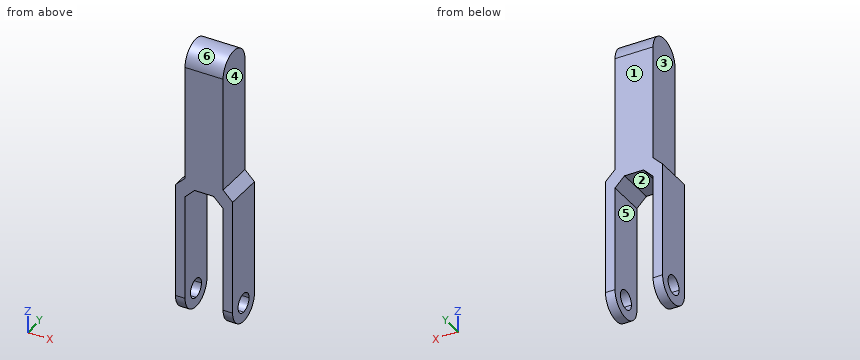
from build123d import *

# Parameters (mm, degrees)
BOSS_EXTRUDE1_DEPTH = 30
SKETCH2_W           = 40
SKETCH2_H           = 20
SKETCH2_W_2         = 10
CUT_EXTRUDE1_DEPTH  = 275.590604355


with BuildPart() as part:
    # Sketch1 → Boss-Extrude1 (new, symmetric)
    with BuildSketch(Plane(origin=(0, 0, 0), x_dir=(0, 0, -1), z_dir=(1, 0, 0))):
        with BuildLine():
            ThreePointArc((20, 0), (14.142135624, 14.142135624), (0, 20))
            Line((0, 20), (0, 10))
            ThreePointArc((0, 10), (7.071067812, 7.071067812), (10, 0))
            ThreePointArc((10, 0), (7.071067812, -7.071067812), (0, -10))
            Line((0, -10), (0, -20))
            ThreePointArc((0, -20), (14.142135624, -14.142135624), (20, 0))
        make_face()
        with BuildLine():
            Line((0, 10), (0, 20))
            ThreePointArc((0, 20), (-20, 0), (0, -20))
            Line((0, -20), (0, -10))
            ThreePointArc((0, -10), (-10, 0), (0, 10))
        make_face()
        with BuildLine():
            ThreePointArc((20, 0), (14.142135624, 14.142135624), (0, 20))
            Line((0, 20), (0, 10))
            ThreePointArc((0, 10), (7.071067812, 7.071067812), (10, 0))
            ThreePointArc((10, 0), (7.071067812, -7.071067812), (0, -10))
            Line((0, -10), (0, -20))
            ThreePointArc((0, -20), (14.142135624, -14.142135624), (20, 0))
        make_face()
        with BuildLine():
            Line((0, 10), (0, 20))
            ThreePointArc((0, 20), (-20, 0), (0, -20))
            Line((0, -20), (0, -10))
            ThreePointArc((0, -10), (-10, 0), (0, 10))
        make_face()
        with BuildLine():
            Line((250, 20), (0, 20))
            ThreePointArc((0, 20), (14.142135624, 14.142135624), (20, 0))
            ThreePointArc((20, 0), (14.142135624, -14.142135624), (0, -20))
            Line((0, -20), (250, -20))
            ThreePointArc((250, -20), (230, 0), (250, 20))
        make_face()
        with BuildLine():
            ThreePointArc((270, 0), (264.142135624, 14.142135624), (250, 20))
            Line((250, 20), (250, 10))
            ThreePointArc((250, 10), (257.071067812, 7.071067812), (260, 0))
            ThreePointArc((260, 0), (257.071067812, -7.071067812), (250, -10))
            Line((250, -10), (250, -20))
            ThreePointArc((250, -20), (264.142135624, -14.142135624), (270, 0))
        make_face()
        with BuildLine():
            Line((250, 10), (250, 20))
            ThreePointArc((250, 20), (230, 0), (250, -20))
            Line((250, -20), (250, -10))
            ThreePointArc((250, -10), (240, 0), (250, 10))
        make_face()
        with BuildLine():
            ThreePointArc((270, 0), (264.142135624, 14.142135624), (250, 20))
            Line((250, 20), (250, 10))
            ThreePointArc((250, 10), (257.071067812, 7.071067812), (260, 0))
            ThreePointArc((260, 0), (257.071067812, -7.071067812), (250, -10))
            Line((250, -10), (250, -20))
            ThreePointArc((250, -20), (264.142135624, -14.142135624), (270, 0))
        make_face()
        with BuildLine():
            Line((250, 10), (250, 20))
            ThreePointArc((250, 20), (230, 0), (250, -20))
            Line((250, -20), (250, -10))
            ThreePointArc((250, -10), (240, 0), (250, 10))
        make_face()
        with BuildLine():
            ThreePointArc((10, 0), (7.071067812, 7.071067812), (0, 10))
            Line((0, 10), (0, -10))
            ThreePointArc((0, -10), (7.071067812, -7.071067812), (10, 0))
        make_face()
        with BuildLine():
            Line((0, -10), (0, 10))
            ThreePointArc((0, 10), (-10, 0), (0, -10))
        make_face()
        with BuildLine():
            ThreePointArc((10, 0), (7.071067812, 7.071067812), (0, 10))
            Line((0, 10), (0, -10))
            ThreePointArc((0, -10), (7.071067812, -7.071067812), (10, 0))
        make_face()
        with BuildLine():
            Line((0, -10), (0, 10))
            ThreePointArc((0, 10), (-10, 0), (0, -10))
        make_face()
    extrude(amount=BOSS_EXTRUDE1_DEPTH, both=True)

    # Sketch2 → Cut-Extrude1 (cut, through all)
    with BuildSketch(Plane(origin=(0, 20, 0), x_dir=(1, 0, 0), z_dir=(0, 1, 0))):
        with Locations((0, 260)):
            Rectangle(SKETCH2_W, SKETCH2_H)
        Polygon((20, 250), (-20, 250), (-20, 140), (-10, 130), (10, 130), (20, 140), align=None)
        Polygon((-20, 120), (-30, 130), (-30, 0), (-20, 0), align=None)
        Polygon((30, 130), (20, 120), (20, 0), (30, 0), align=None)
        with Locations((-25, -10)):
            Rectangle(SKETCH2_W_2, SKETCH2_H)
        with Locations((25, -10)):
            Rectangle(SKETCH2_W_2, SKETCH2_H)
    extrude(amount=-CUT_EXTRUDE1_DEPTH, mode=Mode.SUBTRACT)


solid = part.part
Part model, mm, in its own coordinate system. Face numbers are marked on the shaded views. A direction names the side the tool comes from. Coordinates: 2 decimals unless noted, no trailing zeros. Loops run counter-clockwise (first coordinate to the right, second up) from the corner with the lowest first, then second, coordinate; pieces in that order, holes last. Notation, with made-up numbers: (11.25, -28) -> (60.25, -28) arc R34 cw to (60.25, 10) -> close; hole circle Ø9 at (24, 14.5). An arc over 180 degrees is marked (long way). Use a Markdown table: item, result. Add a question column.
Item 1: Band-saw the part on D-D on z = -185. Write the cut outline in (x, y), plus the area to 3 significant figures.
Item 2: Band-saw the part on A-A on z = -136.5. Write the cut outline in (x, y), plus the area to 3 significant figures.
Item 3: Flat gauge pins, fed straight in: P1, Ø3, axis at x = 19, y = -3.5, coming from the -Z side; P2, Ø1.5, axis at x = -4, y = -6.5, coming from the -Z side; P3, Ø1, axis at x = -2.5, y = -14.5, coming from the +Z side. Where does each tip first touch, or does it go through?
Item 4: Which spindle directions (+Z, -Z, +X, -X, +Y, -Y) get a long thin tool onto all of the face, cutting with end or side? Do the marked faces 5 and 6. Say none if no direction does.
Item 5: Band-saw the part on B-B on y = -14. Write the cut outline in (x, z).
Item 6: Band-saw the part on C-C on x = -5.5. Write the cut outline in (y, z).
Item 7: Pull direction X, two halves, no side cores. Call the marked faces 1, 2, 3 and 4: +X half, -X half, draft (parallel to the pull), parting line (faces both ways), or undercut.
Item 8: Probe probe 1 along X at (y, z) = (13, -251); probe 2 along X at (y, z) = (10, -103); probe 3 along Y at (x, z) = (19.5, 1.5). List the from-to ranges inside material, lowest first.
Geometry says:
| question | item | result |
|---|---|---|
| 1 | outline | (-30, -20) -> (-20, -20) -> (-20, 20) -> (-30, 20) -> close; (20, -20) -> (30, -20) -> (30, 20) -> (20, 20) -> close |
| 1 | area | 800 mm² |
| 2 | outline | (-30, -20) -> (-16.5, -20) -> (-16.5, 20) -> (-30, 20) -> close; (16.5, -20) -> (30, -20) -> (30, 20) -> (16.5, 20) -> close |
| 2 | area | 1,080 mm² |
| 3 | P1 | z = -269.86 |
| 3 | P2 | z = -130 |
| 3 | P3 | z = 14.28 |
| 4 | face 5 | -Z, +Y, -Y |
| 4 | face 6 | +Z, +X, -X |
| 5 | outline | (-30, -264.28) -> (-20, -264.28) -> (-20, -140) -> (-10, -130) -> (10, -130) -> (20, -140) -> (20, -264.28) -> (30, -264.28) -> (30, -130) -> (20, -120) -> (20, 14.28) -> (-20, 14.28) -> (-20, -120) -> (-30, -130) -> close |
| 6 | outline | (-20, -130) -> (20, -130) -> (20, 0) arc R20 ccw to (-20, 0) -> close |
| 7 | face 1 | draft |
| 7 | face 2 | undercut |
| 7 | face 3 | -X half |
| 7 | face 4 | +X half |
| 8 | probe 1 | -30 to -20, 20 to 30 |
| 8 | probe 2 | -20 to 20 |
| 8 | probe 3 | -19.94 to 19.94 |
